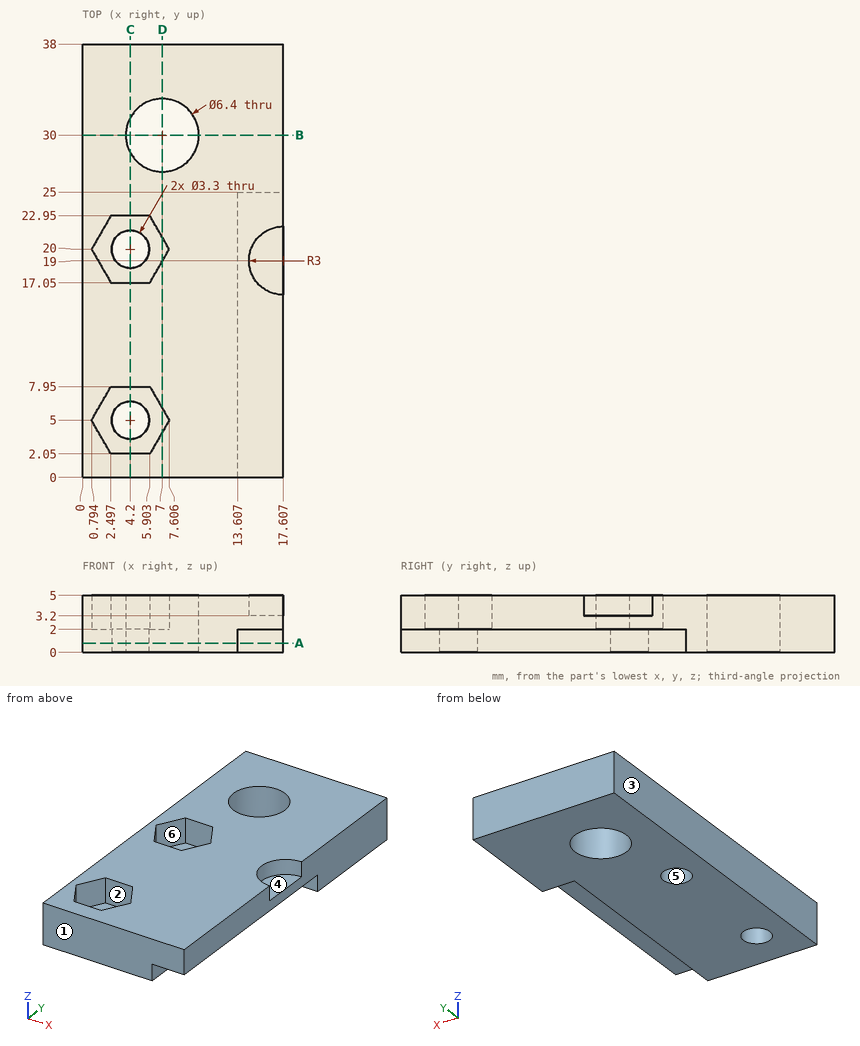
Print and shaded views of the part. All mm, measured from the part's lowest x, y and z. A direction names the side the tool comes from. Coordinates: 2 decimals unless noted, no trailing zeros. Write each loop counter-clockwise with the first axis right and the second up, starting at its lowest first coordinate (ties: lowest second). Pieces come first, ordered by that corner, then holes.
(1) 3-axis set-ups, long thin cutter, end or side, ignore diameter. For the marked faces 4, 5 and 6: which of +Z, -Z, +X, -X, +Y, -Y reach the whole face in a straight line?
(2) Cut at B-B, the plane y = 30. List the corners of the cut face in (x, z).
(3) Cut at D-D, the plane x = 7. List the corners of the cut face in (y, z).
(4) Drill centre lines: probe 1 along X at (y, z) = (5, 0.8); probe 2 along Y at (x, z) = (4.2, 0.55); probe 3 along Y at (x, z) = (4.75, 1.75) (1 decimal). Where is each one in solid material? Low to high.
(5) Cut at A-A, the plane z = 0.8. List the corners of the cut face in (x, y), and give its area (3 significant figures).
(6) Cut at C-C, the plane x = 4.2. List the corners of the cut face in (y, z), and give its area (3 significant figures).
(7) Flat gauge pins, fed straight in: pin 1 (1.8 mm diameter, centred on x = 4, y = 20.5, fed in from +Z); pin 2 (4.5 mm diameter, centred on x = 16, y = 8, fed in from -Z); pin 3 (5.5 mm diameter, centred on x = 4.2, y = 20, fed in from +Z); pin 4 (1 mm diameter, centred on x = 15, z = 0.5, fed in from -Y). Where does each tip first touch, or does it go through?
(8) Two-plate mould, pull along X, no slides. Class the marked faces 1, 2 and 3: +X half, -X half, draft (parallel to the pull), parting line (faces both ways), or undercut.
Geometry says:
1. face 4: +Z, +X
1. face 5: +Z, -Z
1. face 6: +Z
2. outline: (0, 0) - (3.8, 0) - (3.8, 5) - (0, 5) - close; (10.2, 0) - (17.61, 0) - (17.61, 5) - (10.2, 5) - close
3. outline: (0, 0) - (26.8, 0) - (26.8, 5) - (21.05, 5) - (21.05, 2) - (18.95, 2) - (18.95, 5) - (6.05, 5) - (6.05, 2) - (3.95, 2) - (3.95, 5) - (0, 5) - close; (33.2, 0) - (38, 0) - (38, 5) - (33.2, 5) - close
4. probe 1: x = 0 to 2.55, 5.85 to 13.61
4. probe 2: y = 0 to 3.35, 6.65 to 18.35, 21.65 to 28.45, 31.55 to 38
4. probe 3: y = 0 to 3.4, 6.6 to 18.4, 21.6 to 27.7, 32.3 to 38
5. outline: (0, 0) - (13.61, 0) - (13.61, 25) - (17.61, 25) - (17.61, 38) - (0, 38) - close; hole circle Ø3.3 at (4.2, 5); hole circle Ø3.3 at (4.2, 20); hole circle Ø6.4 at (7, 30)
5. area: 520 mm2
6. outline: (0, 0) - (3.35, 0) - (3.35, 2) - (2.05, 2) - (2.05, 5) - (0, 5) - close; (6.65, 0) - (18.35, 0) - (18.35, 2) - (17.05, 2) - (17.05, 5) - (7.95, 5) - (7.95, 2) - (6.65, 2) - close; (21.65, 0) - (28.45, 0) - (28.45, 5) - (22.95, 5) - (22.95, 2) - (21.65, 2) - close; (31.55, 0) - (38, 0) - (38, 5) - (31.55, 5) - close
6. area: 126 mm2
7. pin 1: passes through
7. pin 2: stops at z = 2
7. pin 3: stops at z = 2
7. pin 4: stops at y = 25
8. face 1: draft
8. face 2: undercut
8. face 3: -X half
